For this review, take the finished solid that the model builds, in its own axes (mm). Face numbers are marked on the shaded views. A direction names the side the tool comes from. Give positions to 0.01 mm unless a question says otherwise; leave off trailing zeros. Write each loop counter-clockwise with the first axis right and the second up, starting at its lowest first coordinate (ties: lowest second). Pieces come first, ordered by that corner, then holes. Notation, with made-up numbers: M 71,85 L 100,85 A27 ccw 100,108 Z; hole C -11,63 d1. An arc over 180 degrees is marked long. One line per item, written item: value. Start each with the question number.
Item 1: Consider section D-D, the plane x = -459. Write out the cut boundary in (y, z), and give its area (3 significant figures).
Item 2: To check wall thickness, follow probe 1 along Y at (x, z) = (-48.5, -32.5); probe 2 along Y at (x, z) = (-274, -34.5); probe 3 along Z at (x, y) = (-185, -166.5). State the ranges of each line that lie inside material, in increasing order.
Item 3: Clearance check with flat-ended pins moving along their axes: pin 1 Ø4 at (x, y) = (-420.5, -147) entering from -Z; pin 2 Ø1 at (x, z) = (-180.5, -13.5) entering from +Y; pin 3 Ø10.5 at (x, z) = (-103.5, -14) entering from +Y. State where each tip first meets the part, or that it passes through.
Item 4: Consider section B-B, the plane x = -123. Write out the cut boundary in (y, z), and give its area (3 significant figures).
Item 5: Consider section C-C, the plane y = -167. Write out the cut boundary in (x, z).
Item 6: Consider section A-A, the plane z = -29.5. Write out the cut boundary in (x, y), and give its area (3 significant figures).
Item 7: Tool access review of the marked faces 1, 2 and 3: name each direction out of +Z, -Z, +X, -X, +Y, -Y from which nothing blocks a thin tool from reaching the whole face with its end or side.
```python
from build123d import *

# Parameters (mm, degrees)
BOSS_EXTRUDE1_DEPTH = 6.35
BOSS_EXTRUDE2_DEPTH = 558.8
CUT_EXTRUDE1_START  = -93.726
CUT_EXTRUDE1_DEPTH  = 93.726
CUT_EXTRUDE2_DEPTH  = 93.726
BOSS_EXTRUDE3_DEPTH = 42.164


with BuildPart() as part:
    # Sketch1 → Boss-Extrude1 (new body)
    with BuildSketch(Plane.XY):
        with BuildLine():
            Line((-508.085110878, -46.817945662), (-508.085110878, -168.737945662))
            Line((-508.085110878, -168.737945662), (-508.085110878, -181.437945662))
            ThreePointArc((-508.085110878, -181.437945662), (-500.64562312, -199.398457904), (-482.685110878, -206.837945662))
            Line((-482.685110878, -206.837945662), (50.714889122, -206.837945662))
            Line((50.714889122, -206.837945662), (50.714889122, -21.417945662))
            Line((50.714889122, -21.417945662), (-482.685110878, -21.417945662))
            ThreePointArc((-482.685110878, -21.417945662), (-500.64562312, -28.85743342), (-508.085110878, -46.817945662))
        make_face()
    extrude(amount=BOSS_EXTRUDE1_DEPTH)

    # Sketch2 → Boss-Extrude2 (add, through all)
    with BuildSketch(Plane(origin=(50.714889122, 0, 0), x_dir=(0, 0, -1), z_dir=(1, 0, 0))):
        with BuildLine():
            Line((0, -173.055945662), (0, -206.837945662))
            Line((0, -206.837945662), (2.032, -206.837945662))
            Line((2.032, -206.837945662), (2.032, -194.137945662))
            ThreePointArc((2.032, -194.137945662), (21.082, -175.087945662), (40.132, -194.137945662))
            Line((40.132, -194.137945662), (40.132, -206.837945662))
            Line((40.132, -206.837945662), (42.164, -206.837945662))
            Line((42.164, -206.837945662), (42.164, -194.137945662))
            ThreePointArc((42.164, -194.137945662), (35.989225161, -179.230720501), (21.082, -173.055945662))
            Line((21.082, -173.055945662), (0, -173.055945662))
        make_face()
    extrude(amount=-BOSS_EXTRUDE2_DEPTH)

    # Sketch3 → Cut-Extrude1 (cut)
    with BuildSketch(Plane.XY.offset(CUT_EXTRUDE1_START)):
        with BuildLine():
            Line((-508.085110878, -206.837945662), (-482.685110878, -206.837945662))
            ThreePointArc((-482.685110878, -206.837945662), (-500.64562312, -199.398457904), (-508.085110878, -181.437945662))
            Line((-508.085110878, -181.437945662), (-508.085110878, -206.837945662))
        make_face()
    extrude(amount=CUT_EXTRUDE1_DEPTH, mode=Mode.SUBTRACT)

    # Sketch4 → Cut-Extrude2 (cut)
    with BuildSketch(Plane(origin=(0, 0, 0), x_dir=(-1, 0, 0), z_dir=(0, 0, -1))):
        with BuildLine():
            Line((482.685110878, -21.417945662), (-50.714889122, -21.417945662))
            Line((-50.714889122, -21.417945662), (508.085110878, -107.777945662))
            Line((508.085110878, -107.777945662), (508.085110878, -46.817945662))
            ThreePointArc((508.085110878, -46.817945662), (500.64562312, -28.85743342), (482.685110878, -21.417945662))
        make_face()
    extrude(amount=-CUT_EXTRUDE2_DEPTH, mode=Mode.SUBTRACT)

    # Sketch5 → Boss-Extrude3 (add, through all)
    with BuildSketch(Plane(origin=(0, 0, 0), x_dir=(-1, 0, 0), z_dir=(0, 0, -1))):
        Polygon((-50.714889122, -21.417945662), (508.085110878, -107.777945662), (508.085110878, -110.317945662), (-50.714889122, -23.957945662), align=None)
    extrude(amount=BOSS_EXTRUDE3_DEPTH)


solid = part.part
```
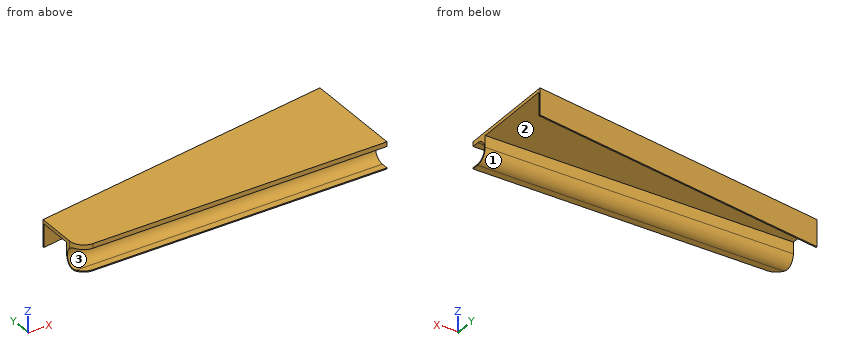
Model answer:
1. outline: M -206.84,-42.16 L -194.14,-42.16 A21.08 ccw -173.06,-21.08 L -173.06,0 L -102.73,0 L -102.73,-42.16 L -100.19,-42.16 L -100.19,6.35 L -206.84,6.35 L -206.84,-2.03 L -194.14,-2.03 A19.05 cw -194.14,-40.13 L -206.84,-40.13 Z
1. area: 1,060 mm2
2. probe 1: y = -178.89 to -176.42, -39.29 to -36.75
2. probe 2: y = -180.62 to -177.88, -74.14 to -71.6
2. probe 3: z = 0 to 6.35
3. pin 1: stops at z = 0
3. pin 2: stops at y = -57.07
3. pin 3: stops at y = -44.44
4. outline: M -206.84,-42.16 L -194.14,-42.16 A21.08 ccw -173.06,-21.08 L -173.06,0 L -50.8,0 L -50.8,-42.16 L -48.26,-42.16 L -48.26,6.35 L -206.84,6.35 L -206.84,-2.03 L -194.14,-2.03 A19.05 cw -194.14,-40.13 L -206.84,-40.13 Z
4. area: 1,390 mm2
5. outline: M -508.09,0 L 50.71,0 L 50.71,6.35 L -508.09,6.35 Z
6. outline: M -508.09,-177.05 L 50.71,-177.05 L 50.71,-174.81 L -508.09,-174.81 Z; M -508.09,-110.32 L 50.71,-23.96 L 50.71,-21.42 L -508.09,-107.78 Z
6. area: 2,670 mm2
7. face 1: -Z, +X, -X
7. face 2: -Z, +X
7. face 3: +X, -X, -Y
